```python
from build123d import *

# Parameters (mm, degrees)
F0_W     = 48
F0_H     = 15
F1_DEPTH = 12
F2_W     = 42.5
F2_H     = 10.5
F3_DEPTH = 7
F4_R     = 1.75
F5_DEPTH = 5


# Not quite as in the source:
# - a pattern or mirror of a feature is missing from the dataset's text; its kind, count and spacing are read off the source's solid


with BuildPart() as f1:
    # F0 (on Front) → F1 (new body)
    with BuildSketch(Plane.XZ):
        Rectangle(F0_W, F0_H)
    extrude(amount=F1_DEPTH)

    # F2 (on face) → F3 (cut)
    with BuildSketch(Plane.XZ.offset(12)):
        Rectangle(F2_W, F2_H)
    extrude(amount=-F3_DEPTH, mode=Mode.SUBTRACT)

    # F4 (on face) → F5 (cut, through all)
    with BuildSketch(Plane.XZ.offset(5)):
        with Locations((-15, 0)):
            Circle(F4_R)
    f5 = extrude(amount=-F5_DEPTH, mode=Mode.SUBTRACT)

    # F5_copies: F5 across plane
    add(f5.mirror(Plane(origin=(0, 0, 0), x_dir=(0, 0, 1), z_dir=(1, 0, 0))), mode=Mode.SUBTRACT)


solid = f1.part
```
Geometry check sheet. Reference: the model listing, model coordinates, mm. A direction names the side the tool comes from. Round coordinates to 2 decimals unless told otherwise and drop trailing zeros. Order: outer loops, then holes, each group sorted by start corner. A loop starts at its lowest first (then second) coordinate and runs counter-clockwise, first axis right, second up. Notation, with made-up numbers: M -16,46.5 L 12,46.5 A14 ccw 12,50.5 Z; hole C 88,-9.75 d11. An arc over 180 degrees is marked long. Write item = value, one per line.
Q1. Section check A-A (y = -11). Enter the section's corners in (x, z), plus the area to 3 significant figures.
Answer block:
outline = M -24,-7.5 L 24,-7.5 L 24,7.5 L -24,7.5 Z; hole M -21.25,-5.25 L 21.25,-5.25 L 21.25,5.25 L -21.25,5.25 Z
area = 274 mm^2
Q2. Depth check by flat-ended pin: pin 1 Ø1 at (x, z) = (-4.5, -1) entering from -Y. Enter the tip coordinate at first touch or a pass-through.
Answer block:
pin_1 = -5
Q3. Section check C-C (x = 15). Enter the section's corners in (y, z), plus the area to 3 significant figures.
Answer block:
outline = M -12,-7.5 L 0,-7.5 L 0,-1.75 L -5,-1.75 L -5,-5.25 L -12,-5.25 Z; M -12,5.25 L -5,5.25 L -5,1.75 L 0,1.75 L 0,7.5 L -12,7.5 Z
area = 89.0 mm^2
Q4. Section check D-D (z = -4.75). Enter the section's corners in (x, y).
Answer block:
outline = M -24,-12 L -21.25,-12 L -21.25,-5 L 21.25,-5 L 21.25,-12 L 24,-12 L 24,0 L -24,0 Z
Q5. Scan lines: line 1 (Z direction, x = 15, y = -2.15); line 2 (Z direction, x = -10, y = -10.25); line 3 (X direction, y = -5.5, z = -0.75). Record each from-to range of solid material in increasing order.
Answer block:
line_1 = -7.5 to -1.75, 1.75 to 7.5
line_2 = -7.5 to -5.25, 5.25 to 7.5
line_3 = -24 to -21.25, 21.25 to 24
Q6. Release check for a two-part mould opening along Z. For faces 1 (the flat face through (0, -5, 0)), 2 (the flat face through (0, -6, 7.5)), 3 (the flat face through (24, -6, 0)), 4 (the flat face through (0, -6, -7.5)) record: released by +Z, released by -Z, zero draft, split by the parting line, or undercut.
Answer block:
face_1 = undercut
face_2 = released by +Z
face_3 = zero draft
face_4 = released by -Z
Q7. Set-up check for faces 5 (the flat face through (0, -9, -5.25)), 6 (the flat face through (0, 0, 0)): record each of +Z, -Z, +X, -X, +Y, -Y from which the full face is reachable in a straight line by a thin tool's end or side.
Answer block:
face_5 = -Y
face_6 = +Z, -Z, +X, -X, +Y
Q8. Section check B-B (z = 0). Enter the section's corners in (x, y).
Answer block:
outline = M -24,-12 L -21.25,-12 L -21.25,-5 L -16.75,-5 L -16.75,0 L -24,0 Z; M -13.25,-5 L 13.25,-5 L 13.25,0 L -13.25,0 Z; M 16.75,-5 L 21.25,-5 L 21.25,-12 L 24,-12 L 24,0 L 16.75,0 Z
